from build123d import *

# Parameters (mm, degrees)
SKETCH1_R           = 13.25
SKETCH1_R_2         = 2.05
BOSS_EXTRUDE1_DEPTH = 2
SKETCH2_R           = 2
BOSS_EXTRUDE2_DEPTH = 2
BOSS_EXTRUDE3_DEPTH = 2
BOSS_EXTRUDE4_DEPTH = 2
SKETCH6_W           = 10
SKETCH6_H           = 5
CUT_EXTRUDE2_DEPTH  = 2
FILLET1_R           = 3
FILLET_1_R          = 2
FILLET_2_R          = 3


with BuildPart() as part:
    # Sketch1 → Boss-Extrude1 (new body)
    with BuildSketch(Plane(origin=(0, 0, 0), x_dir=(0, 0, -1), z_dir=(1, 0, 0))):
        with BuildLine():
            Line((-13, 21.5), (13, 21.5))
            ThreePointArc((13, 21.5), (20.071067812, 18.571067812), (23, 11.5))
            Line((23, 11.5), (23, -21.5))
            Line((23, -21.5), (-23, -21.5))
            Line((-23, -21.5), (-23, 11.5))
            ThreePointArc((-23, 11.5), (-20.071067812, 18.571067812), (-13, 21.5))
        make_face()
        Circle(SKETCH1_R, mode=Mode.SUBTRACT)
        with Locations((0, 17.5)):
            Circle(SKETCH1_R_2, mode=Mode.SUBTRACT)
        with Locations((17.5, 0)):
            Circle(SKETCH1_R_2, mode=Mode.SUBTRACT)
        with Locations((0, -17.5)):
            Circle(SKETCH1_R_2, mode=Mode.SUBTRACT)
        with Locations((-17.5, 0)):
            Circle(SKETCH1_R_2, mode=Mode.SUBTRACT)
    extrude(amount=BOSS_EXTRUDE1_DEPTH)

    # Sketch2 → Boss-Extrude2 (add)
    # profile 1 of 2: a face of its own
    with BuildSketch(Plane.XZ.offset(21.5)):
        Polygon((-12.5, 23), (-12.5, 47), (-2.5, 47), (-2.5, 28), (2, 28), (2, 23), (0, 23), (0, 15), (-12.5, 15), align=None)
        with Locations(Location((-7.5, 33, 0), (0, 0, 90))):
            Circle(SKETCH2_R, mode=Mode.SUBTRACT)
    # profile 2 of 2: a face of its own
    with BuildSketch(Plane.XZ.offset(21.5)):
        Polygon((2, -23), (0, -23), (0, -15), (-12.5, -15), (-12.5, -23), (-12.5, -47), (-2.5, -47), (-2.5, -28), (2, -28), align=None)
        with Locations(Location((-7.5, -33, 0), (0, 0, 270))):
            Circle(SKETCH2_R, mode=Mode.SUBTRACT)
    extrude(amount=-BOSS_EXTRUDE2_DEPTH)

    # Sketch3 → Boss-Extrude3 (add)
    with BuildSketch(Plane(origin=(0, 0, -23), x_dir=(-1, 0, 0), z_dir=(0, 0, -1))):
        Polygon((-2, 11.5), (0, 11.5), (12.5, -19.5), (7.5, -19.5), (-2, -19.55), align=None)
    extrude(amount=BOSS_EXTRUDE3_DEPTH)

    # Sketch4 → Boss-Extrude4 (add)
    with BuildSketch(Plane.XY.offset(23)):
        Polygon((2, 11.5), (0, 11.5), (-12.5, -19.5), (2, -19.5), align=None)
    extrude(amount=BOSS_EXTRUDE4_DEPTH)

    # Sketch6 → Cut-Extrude2 (cut)
    with BuildSketch(Plane(origin=(0, -19.5, 0), x_dir=(1, 0, 0), z_dir=(0, 1, 0))):
        with Locations((-7.5, 44.5)):
            Rectangle(SKETCH6_W, SKETCH6_H)
        with Locations((-7.5, -44.5)):
            Rectangle(SKETCH6_W, SKETCH6_H)
    extrude(amount=-CUT_EXTRUDE2_DEPTH, mode=Mode.SUBTRACT)

    # Fillet1
    fillet1_edges = [part.edges().sort_by_distance(p)[0] for p in [
        (-2.5, -20.5, -42),
        (-12.5, -20.5, -42),
        (-12.5, -20.5, 42),
        (-2.5, -20.5, 42),
    ]]
    fillet(fillet1_edges, radius=FILLET1_R)

    # 圆角1
    fillet_1_edges = [part.edges().sort_by_distance(p)[0] for p in [
        (2, -20.5, -28),
        (-2.5, -20.5, -28),
        (-2.5, -20.5, 28),
        (2, -20.5, 28),
    ]]
    fillet(fillet_1_edges, radius=FILLET_1_R)

    # 圆角2
    fillet_2_edges = [part.edges().sort_by_distance(p)[0] for p in [
        (-12.5, -20.5, -15),
        (-12.5, -20.5, 15),
    ]]
    fillet(fillet_2_edges, radius=FILLET_2_R)


solid = part.part
The listing builds one solid part. Answer for the finished solid, in the listing's coordinates (mm). A direction names the side the tool comes from. Coordinates: 2 decimals unless noted, no trailing zeros. Write each loop counter-clockwise with the first axis right and the second up, starting at its lowest first coordinate (ties: lowest second). Pieces come first, ordered by that corner, then holes. Notation, with made-up numbers: (-31.5, 79) - (-7.5, 79) arc R36 ccw to (-7.5, 118) - close; hole circle Ø7 at (-34.5, 82). An arc over 180 degrees is marked (long way). Answer as CSV lines item,"result".
1. Find section A-A (z = 0). Give the vertices of the cut face in (x, y).
Computed values:
outline,"(0, -21.5) - (2, -21.5) - (2, -19.55) - (0, -19.55) - close; (0, -15.45) - (2, -15.45) - (2, -13.25) - (0, -13.25) - close; (0, 13.25) - (2, 13.25) - (2, 15.45) - (0, 15.45) - close; (0, 19.55) - (2, 19.55) - (2, 21.5) - (0, 21.5) - close"
2. Determine the mould class of faces 1 (the flat face through (-12.5, -21, 29)), 2 (the cylindrical face through (0.99, 0.09, -15.45)), 3 (the flat face through (1, 11.5, 24)) for opening direction Y: +Y half, -Y half, draft (parallel to the pull), parting line (faces both ways), or undercut.
Computed values:
face 1,"draft"
face 2,"undercut"
face 3,"+Y half"
3. Find section B-B (x = -7.5). Give the vertices of the cut face in (y, z), plus the area to 3 significant figures.
Computed values:
outline,"(-21.5, -42) - (-19.5, -42) - (-19.5, -35) - (-21.5, -35) - close; (-21.5, -31) - (-19.5, -31) - (-19.5, -25) - (-7.1, -25) - (-7.1, -23) - (-19.5, -23) - (-19.5, -15) - (-21.5, -15) - close; (-21.5, 15) - (-19.5, 15) - (-19.5, 23) - (-7.1, 23) - (-7.1, 25) - (-19.5, 25) - (-19.5, 31) - (-21.5, 31) - close; (-21.5, 35) - (-19.5, 35) - (-19.5, 42) - (-21.5, 42) - close"
area,"142 mm²"
4. Given P1, Ø2.5, axis at x = -4.5, z = 20, coming from the +Y side; P2, Ø2, axis at x = -3, y = 2.5, coming from the -Z side; P3, Ø4.5, axis at y = 0, z = -17.5, coming from the -X side, each flat-ended and moving along its own axis, determine where each tip first touches the part or whether it passes through.
Computed values:
P1,"stops at y = -19.5"
P2,"stops at z = -25"
P3,"stops at x = 0"
5. A tool of negligible diameter and unlimited length cuts with its end or side. For faces 4 (the flat face through (-5, -19.5, -33)), 5 (the cylindrical face through (-11.64, -20.49, -15.9)), 6 (the flat face through (-4, -11, -23)), from which of +Z, -Z, +X, -X, +Y, -Y can it reach the whole face along a straight path? Write none if from no direction.
Computed values:
face 4,"-Z, +X, -X, +Y"
face 5,"-X, +Y, -Y"
face 6,"-X, +Y"
6. Find section C-C (y = 17.5). Give the vertices of the cut face in (x, z), plus the area to 3 significant figures.
Computed values:
outline,"(0, -21) - (2, -21) - (2, -2.05) - (0, -2.05) - close; (0, 2.05) - (2, 2.05) - (2, 21) - (0, 21) - close"
area,"75.8 mm²"
7. Find section D-D (z = 33). Give the vertices of the cut face in (x, y).
Computed values:
outline,"(-12.5, -21.5) - (-9.5, -21.5) - (-9.5, -19.5) - (-12.5, -19.5) - close; (-5.5, -21.5) - (-2.5, -21.5) - (-2.5, -19.5) - (-5.5, -19.5) - close"
8. Straight lines are drawn through the part: line 1 (Y direction, x = 0.75, z = 0); line 2 (Z direction, x = -4, y = -4); line 3 (X direction, y = -20.25, z = 33). For each, find the intervals that lie inside material, in ascending order. Write a range as [from, to].
Computed values:
line 1,"y = [-21.5, -19.55], [-15.45, -13.25], [13.25, 15.45], [19.55, 21.5]"
line 2,"z = [-25, -23], [23, 25]"
line 3,"x = [-12.5, -9.5], [-5.5, -2.5]"
